Read the model definition and answer for the solid it produces. Units are mm, in the model's axes. A direction names the side the tool comes from. Round coordinates to 2 decimals unless told otherwise and drop trailing zeros. Loops run counter-clockwise (first coordinate to the right, second up) from the corner with the lowest first, then second, coordinate; pieces in that order, holes last. Notation, with made-up numbers: (-40, 24.5) - (-25, 24.5) arc R21 ccw to (-25, 52.5) - close; hole circle Ø8 at (-34, -36). An arc over 180 degrees is marked (long way). Answer as CSV lines item,"result".
```python
from build123d import *

# Parameters (mm, degrees)
SKETCH_1_R          = 55
EXTRUDE_1_DEPTH     = 60
SKETCH_2_R          = 50
CUT_EXTRUDE_1_DEPTH = 47
SKETCH_3_R          = 17
CUT_EXTRUDE_2_DEPTH = 14
SKETCH_4_R          = 4
CUT_EXTRUDE_3_DEPTH = 61
SKETCH1_R           = 21.1
CUT_EXTRUDE1_DEPTH  = 8
CHAMFER1_SIZE       = 1
CHAMFER1_SIZE2      = 1.732050808
SKETCH2_R           = 2
CUT_EXTRUDE2_DEPTH  = 61
CUT_EXTRUDE3_DEPTH  = 4


with BuildPart() as part:
    # Эскиз1 → Бобышка-Вытянуть1 (new body)
    with BuildSketch(Plane(origin=(0, 0, 0), x_dir=(1, 0, 0), z_dir=(0, 1, 0))):
        with Locations(Location((0, 0, 0), (0, 0, 270))):  # turned: the seam where the file's is
            Circle(SKETCH_1_R)
    extrude(amount=EXTRUDE_1_DEPTH)

    # Эскиз2 → Вырез-Вытянуть1 (cut)
    with BuildSketch(Plane.XZ):
        with Locations(Location((0, 0, 0), (0, 0, 270))):  # turned: the seam where the file's is
            Circle(SKETCH_2_R)
    extrude(amount=-CUT_EXTRUDE_1_DEPTH, mode=Mode.SUBTRACT)

    # Эскиз3 → Вырез-Вытянуть2 (cut, through all)
    with BuildSketch(Plane.XZ.offset(-47)):
        with Locations(Location((0, 0, 0), (0, 0, 270))):  # turned: the seam where the file's is
            Circle(SKETCH_3_R)
    extrude(amount=-CUT_EXTRUDE_2_DEPTH, mode=Mode.SUBTRACT)

    # Эскиз4 → Вырез-Вытянуть3 (cut, through all)
    with BuildSketch(Plane(origin=(0, 60, 0), x_dir=(1, 0, 0), z_dir=(0, 1, 0))):
        with Locations(Location((33.591727056, -32.872418125, 0), (0, 0, 270))):  # turned: the seam where the file's is
            Circle(SKETCH_4_R)
        with Locations(Location((-33.591727056, -32.872418125, 0), (0, 0, 270))):  # turned: the seam where the file's is
            Circle(SKETCH_4_R)
        with Locations(Location((-33.591727056, 32.872418125, 0), (0, 0, 270))):  # turned: the seam where the file's is
            Circle(SKETCH_4_R)
        with Locations(Location((33.591727056, 32.872418125, 0), (0, 0, 270))):  # turned: the seam where the file's is
            Circle(SKETCH_4_R)
    extrude(amount=-CUT_EXTRUDE_3_DEPTH, mode=Mode.SUBTRACT)

    # Sketch1 → Cut-Extrude1 (cut)
    with BuildSketch(Plane(origin=(0, 60, 0), x_dir=(1, 0, 0), z_dir=(0, 1, 0))):
        with Locations(Location((0, 0, 0), (0, 0, 270))):  # turned: the seam where the file's is
            Circle(SKETCH1_R)
    extrude(amount=-CUT_EXTRUDE1_DEPTH, mode=Mode.SUBTRACT)

    # Chamfer1
    chamfer1_edges = [part.edges().sort_by_distance(p)[0] for p in [
        (0, 60, -21.1),
    ]]
    chamfer1_side = [part.faces().sort_by_distance(p)[0] for p in [
        (0, 60, -53.444365081),
    ]]
    chamfer(chamfer1_edges, length=CHAMFER1_SIZE, length2=CHAMFER1_SIZE2, reference=chamfer1_side[0])

    # Sketch2 → Cut-Extrude2 (cut, through all)
    with BuildSketch(Plane(origin=(0, 60, 0), x_dir=(1, 0, 0), z_dir=(0, 1, 0))):
        with Locations(Location((21, 21, 0), (0, 0, 270))):  # turned: the seam where the file's is
            Circle(SKETCH2_R)
        with Locations(Location((-21, 21, 0), (0, 0, 270))):  # turned: the seam where the file's is
            Circle(SKETCH2_R)
        with Locations(Location((21, -21, 0), (0, 0, 270))):  # turned: the seam where the file's is
            Circle(SKETCH2_R)
        with Locations(Location((-21, -21, 0), (0, 0, 270))):  # turned: the seam where the file's is
            Circle(SKETCH2_R)
    extrude(amount=-CUT_EXTRUDE2_DEPTH, mode=Mode.SUBTRACT)

    # Sketch3 → Cut-Extrude3 (cut)
    with BuildSketch(Plane.XZ.offset(-47)):
        Polygon((-21, -16.9), (-24.550704156, -18.95), (-24.550704156, -23.05), (-21, -25.1), (-17.449295844, -23.05), (-17.449295844, -18.95), align=None)
        Polygon((-21, 25.1), (-24.550704156, 23.05), (-24.550704156, 18.95), (-21, 16.9), (-17.449295844, 18.95), (-17.449295844, 23.05), align=None)
        Polygon((24.550704156, 23.05), (21, 25.1), (17.449295844, 23.05), (17.449295844, 18.95), (21, 16.9), (24.550704156, 18.95), align=None)
        Polygon((24.550704156, -18.95), (21, -16.9), (17.449295844, -18.95), (17.449295844, -23.05), (21, -25.1), (24.550704156, -23.05), align=None)
    extrude(amount=-CUT_EXTRUDE3_DEPTH, mode=Mode.SUBTRACT)


solid = part.part
```
1) The mould has two halves that part along Z. Classify faces 1 (the face through (22.75, 48.97, 17.91)), 2 (the face through (-49.997, 23.171, 0.504)): pulls with the +Z half, pulls with the -Z half, needs draft (parallel to the pull), parting line crosses it, or undercut.
Entries:
face 1,"undercut"
face 2,"undercut"
2) Find the intervals of material crossed by line 1 (Y direction, x = 15, z = 35); line 2 (Z direction, x = -17, y = 20.5); line 3 (X direction, y = 7, z = -7.5), in increasing order.
Entries:
line 1,"y = 47 to 60"
line 2,"z = -52.31 to -47.02, 47.02 to 52.31"
line 3,"x = -54.49 to -49.43, 49.43 to 54.49"
3) A tool of negligible diameter and unlimited length cuts with its end or side. For faces 3 (the face through (17.3, 52, 1.5)), 4 (the face through (-37.14, 43.75, 34.72)), 5 (the face through (19.2, 48.97, 17.94)), from which of +Z, -Z, +X, -X, +Y, -Y can it reach the whole face along a straight path? Write none if from no direction.
Entries:
face 3,"+Y"
face 4,"+Y, -Y"
face 5,"-Y"
4) A cutting plane is placed at D-D, the plane x = -32. Determine the outline of the cut face in (y, z), plus the area to 3 significant figures.
Entries:
outline,"(0, -44.73) - (60, -44.73) - (60, -36.54) - (47, -36.54) - (47, -38.42) - (0, -38.42) - close; (0, 38.42) - (47, 38.42) - (47, 36.54) - (60, 36.54) - (60, 44.73) - (0, 44.73) - close; (47, -29.2) - (60, -29.2) - (60, 29.2) - (47, 29.2) - close"
area,"1,570 mm^2"
5) A cutting plane is placed at C-C, the plane y = 31.5. Determine the outline of the cut face in (x, z), plus the area to 3 significant figures.
Entries:
outline,"circle Ø110 at (0, 0); hole (-37.59, -32.97) arc R4 ccw to (-33.77, -36.87) arc R50 ccw to (33.77, -36.87) arc R4 ccw to (37.59, -32.97) arc R50 ccw to (37.59, 32.97) arc R4 ccw to (33.77, 36.87) arc R50 ccw to (-33.77, 36.87) arc R4 ccw to (-37.59, 32.97) arc R50 ccw to start"
area,"1,630 mm^2"
6) A cutting plane is placed at B-B, the plane x = 0. Determine the outline of the cut face in (y, z), plus the area to 3 significant figures.
Entries:
outline,"(0, -55) - (60, -55) - (60, -22.1) - (58.27, -21.1) - (52, -21.1) - (52, -17) - (47, -17) - (47, -50) - (0, -50) - close; (0, 50) - (47, 50) - (47, 17) - (52, 17) - (52, 21.1) - (58.27, 21.1) - (60, 22.1) - (60, 55) - (0, 55) - close"
area,"1,390 mm^2"
7) Each of these flat-tipped pins is pushed along its axis until it touches: P1, Ø4.5, axis at y = 48.5, z = -21.5, coming from the +X side; P2, Ø2.5, axis at x = 21, z = 21, coming from the +Y side; P3, Ø1, axis at x = 2, z = -38.5, coming from the -Y side; P4, Ø6, axis at y = 27, z = 25.5, coming from the +X side. Where does it stop, or does it pass through?
Entries:
P1,"stops at x = 51.52"
P2,"passes through"
P3,"stops at y = 47"
P4,"stops at x = 50.19"
8) A cutting plane is placed at A-A, the plane z = 0. Determine the outline of the cut face in (x, y), plus the area to 3 significant figures.
Entries:
outline,"(-55, 0) - (-50, 0) - (-50, 47) - (-17, 47) - (-17, 52) - (-21.1, 52) - (-21.1, 58.27) - (-22.1, 60) - (-55, 60) - close; (17, 47) - (50, 47) - (50, 0) - (55, 0) - (55, 60) - (22.1, 60) - (21.1, 58.27) - (21.1, 52) - (17, 52) - close"
area,"1,390 mm^2"
